from build123d import *

# Parameters (mm, degrees)
SKETCH1_W           = 20
SKETCH1_H           = 190
SKETCH1_R           = 1.6
SKETCH1_R_2         = 7
BOSS_EXTRUDE1_DEPTH = 3.175
FILLET1_R           = 3
FILLET2_R           = 8


with BuildPart() as part:
    # Sketch1 → Boss-Extrude1 (new body)
    with BuildSketch(Plane.XY):
        Rectangle(SKETCH1_W, SKETCH1_H)
        with Locations((0, -91)):
            Circle(SKETCH1_R, mode=Mode.SUBTRACT)
        with Locations((0, -79)):
            Circle(SKETCH1_R, mode=Mode.SUBTRACT)
        with Locations((0, -67)):
            Circle(SKETCH1_R, mode=Mode.SUBTRACT)
        with Locations((0, -55)):
            Circle(SKETCH1_R, mode=Mode.SUBTRACT)
        with Locations((0, -43)):
            Circle(SKETCH1_R, mode=Mode.SUBTRACT)
        with Locations((0, -31)):
            Circle(SKETCH1_R, mode=Mode.SUBTRACT)
        with Locations((0, -19)):
            Circle(SKETCH1_R, mode=Mode.SUBTRACT)
        with Locations((0, 85)):
            Circle(SKETCH1_R_2, mode=Mode.SUBTRACT)
        with Locations((0, -7)):
            Circle(SKETCH1_R, mode=Mode.SUBTRACT)
        with Locations((0, 5)):
            Circle(SKETCH1_R, mode=Mode.SUBTRACT)
        with Locations((0, 17)):
            Circle(SKETCH1_R, mode=Mode.SUBTRACT)
        with Locations((0, 29)):
            Circle(SKETCH1_R, mode=Mode.SUBTRACT)
        with Locations((0, 41)):
            Circle(SKETCH1_R, mode=Mode.SUBTRACT)
        with Locations((0, 53)):
            Circle(SKETCH1_R, mode=Mode.SUBTRACT)
        with Locations((0, 65)):
            Circle(SKETCH1_R, mode=Mode.SUBTRACT)
    extrude(amount=BOSS_EXTRUDE1_DEPTH)

    # Fillet1
    fillet1_edges = [part.edges().sort_by_distance(p)[0] for p in [
        (10, -95, 1.5875),
        (-10, -95, 1.5875),
    ]]
    fillet(fillet1_edges, radius=FILLET1_R)

    # Fillet2
    fillet2_edges = [part.edges().sort_by_distance(p)[0] for p in [
        (-10, 95, 1.5875),
        (10, 95, 1.5875),
    ]]
    fillet(fillet2_edges, radius=FILLET2_R)


solid = part.part
Geometry: final body of the model. Coordinates: model frame, mm. Coordinates: 2 decimals unless noted, no trailing zeros. Order: outer loops, then holes, each group sorted by start corner. A loop starts at its lowest first (then second) coordinate and runs counter-clockwise, first axis right, second up.
(1) Section query A-A (z = 0.65). State how many separate pieces and enclosed holes the cut face has, plus the area to 3 significant figures.
(2) Material intervals for probe 1 along X at (y, z) = (-67, 0.7); probe 2 along Y at (x, z) = (-4, 1.1); probe 3 along Y at (x, z) = (5.25, 1.6), sorted ascending.
(3) Section query C-C (x = -4). Return the cut outline in (y, z) (3 decimals).
(4) Section query B-B (y = 5). Return the cut outline in (x, z) (3 decimals).
(5) Draft query along Y for faces 1 (the face through (-0.208, -17.414, 1.565)), 2 (the face through (-9.14, -94.1, 1.61)), 3 (the face through (0.86, -53.65, 1.57)), 4 (the face through (0, 1, 0)). Return one class per face: pulls with the +Y half, pulls with the -Y half, needs draft (parallel to the pull), parting line crosses it, or undercut.
Solution:
1. separate pieces: 1
1. enclosed holes: 15
1. area: 3,500 mm2
2. probe 1: x = -10 to -1.6, 1.6 to 10
2. probe 2: y = -95 to 79.26, 90.74 to 94.75
2. probe 3: y = -95 to 80.37, 89.63 to 94.31
3. outline: (-95, 0) - (79.255, 0) - (79.255, 3.175) - (-95, 3.175) - close; (90.745, 0) - (94.746, 0) - (94.746, 3.175) - (90.745, 3.175) - close
4. outline: (-10, 0) - (-1.6, 0) - (-1.6, 3.175) - (-10, 3.175) - close; (1.6, 0) - (10, 0) - (10, 3.175) - (1.6, 3.175) - close
5. face 1: undercut
5. face 2: pulls with the -Y half
5. face 3: undercut
5. face 4: needs draft
